Design review of the part built by this model. Coordinates are the model's own, in mm. Give positions to 0.01 mm unless a question says otherwise; leave off trailing zeros. Write each loop counter-clockwise with the first axis right and the second up, starting at its lowest first coordinate (ties: lowest second). Pieces come first, ordered by that corner, then holes. Notation, with made-up numbers: M 71,-26.5 L 75,-26.5 A25 cw 75,0.5 Z; hole C 10,73 d11. An arc over 180 degrees is marked long. Write each question's results on one line, items separated by ' | '. Start each with the question number.
from build123d import *

# Parameters (mm, degrees)
SKETCH1_R                    = 152.9969
SKETCH1_R_2                  = 123.825
BOSS_EXTRUDE1_DEPTH          = 22.352
SKETCH2_R                    = 127.254
CUT_EXTRUDE1_DEPTH           = 11.938
CHAMFER1_SIZE                = 0.762
SKETCH3_R                    = 4.2164
CUT_EXTRUDE2_DEPTH           = 23.352
CHAMFER2_SIZE                = 0.381
CIRPATTERN1_COUNT            = 32
CHAMFER2_OF_CIRPATTERN1_SIZE = 0.381
CUT_EXTRUDE3_DEPTH           = 0.79375


with BuildPart() as part:
    # Sketch1 → Boss-Extrude1 (new body)
    with BuildSketch(Plane(origin=(0, 0, 0), x_dir=(1, 0, 0), z_dir=(0, 1, 0))):
        Circle(SKETCH1_R)
        Circle(SKETCH1_R_2, mode=Mode.SUBTRACT)
    extrude(amount=BOSS_EXTRUDE1_DEPTH)

    # Sketch2 → Cut-Extrude1 (cut)
    with BuildSketch(Plane(origin=(0, 22.352, 0), x_dir=(-1, 0, 0), z_dir=(0, -1, 0))):
        Circle(SKETCH2_R)
    extrude(amount=CUT_EXTRUDE1_DEPTH, mode=Mode.SUBTRACT)

    # Chamfer1
    chamfer1_edges = [part.edges().sort_by_distance(p)[0] for p in [
        (127.254, 22.352, 0),
        (-152.9969, 0, 0),
        (-152.9969, 22.352, 0),
    ]]
    chamfer(chamfer1_edges, length=CHAMFER1_SIZE)

    # Sketch4 → Cut-Revolve1 (revolve, cut)
    with BuildSketch(Plane.XY):
        Polygon((-137.16, 0), (-137.16, 1.6256), (-134.366, 0.6604), (-134.366, 1.27), (0, 1.27), (0, 0), align=None)
    revolve(axis=Axis((0, 22.352, 0), (0, -1, 0)), mode=Mode.SUBTRACT)

    # Sketch3 → Cut-Extrude2 (cut, through all)
    with BuildSketch(Plane(origin=(0, 22.352, 0), x_dir=(1, 0, 0), z_dir=(0, 1, 0))):
        with Locations((-13.918306505, 141.314937447)):
            Circle(SKETCH3_R)
    cut_extrude2 = extrude(amount=-CUT_EXTRUDE2_DEPTH, mode=Mode.SUBTRACT)

    # Chamfer2
    chamfer2_edges = [part.edges().sort_by_distance(p)[0] for p in [
        (-18.134706505, 0, -141.314937447),
        (-18.134706505, 22.352, -141.314937447),
    ]]
    chamfer(chamfer2_edges, length=CHAMFER2_SIZE)

    # CirPattern1: Cut-Extrude2 ×32 about axis
    cirpattern1_axis = Axis((0, 0, 0), (0, 1, 0))
    for i in range(1, CIRPATTERN1_COUNT):
        add(cut_extrude2.rotate(cirpattern1_axis, i * 360 / CIRPATTERN1_COUNT), mode=Mode.SUBTRACT)

    # Chamfer2 of CirPattern1
    chamfer2_of_cirpattern1_edges = [part.edges().sort_by_distance(p)[0] for p in [
        (-45.355429856, 0, -135.061704818),
        (-45.355429856, 22.352, -135.061704818),
        (-70.833169474, 0, -123.618126616),
        (-70.833169474, 22.352, -123.618126616),
        (-93.588830113, 0, -107.423973133),
        (-93.588830113, 22.352, -107.423973133),
        (-112.747924496, 0, -87.101576608),
        (-112.747924496, 22.352, -87.101576608),
        (-127.57417937, 0, -63.43191534),
        (-127.57417937, 22.352, -63.43191534),
        (-137.497830076, 0, -37.324601139),
        (-137.497830076, 22.352, -37.324601139),
        (-142.137516281, 0, -9.782923448),
        (-142.137516281, 22.352, -9.782923448),
        (-141.314937447, 0, 18.134706505),
        (-141.314937447, 22.352, 18.134706505),
        (-135.061704818, 0, 45.355429856),
        (-135.061704818, 22.352, 45.355429856),
        (-123.618126616, 0, 70.833169474),
        (-123.618126616, 22.352, 70.833169474),
        (-107.423973133, 0, 93.588830113),
        (-107.423973133, 22.352, 93.588830113),
        (-87.101576608, 0, 112.747924496),
        (-87.101576608, 22.352, 112.747924496),
        (-63.43191534, 0, 127.57417937),
        (-63.43191534, 22.352, 127.57417937),
        (-37.324601139, 0, 137.497830076),
        (-37.324601139, 22.352, 137.497830076),
        (-9.782923448, 0, 142.137516281),
        (-9.782923448, 22.352, 142.137516281),
        (18.134706505, 0, 141.314937447),
        (18.134706505, 22.352, 141.314937447),
        (45.355429856, 0, 135.061704818),
        (45.355429856, 22.352, 135.061704818),
        (70.833169474, 0, 123.618126616),
        (70.833169474, 22.352, 123.618126616),
        (93.588830113, 0, 107.423973133),
        (93.588830113, 22.352, 107.423973133),
        (112.747924496, 0, 87.101576608),
        (112.747924496, 22.352, 87.101576608),
        (127.57417937, 0, 63.43191534),
        (127.57417937, 22.352, 63.43191534),
        (137.497830076, 0, 37.324601139),
        (137.497830076, 22.352, 37.324601139),
        (142.137516281, 0, 9.782923448),
        (142.137516281, 22.352, 9.782923448),
        (141.314937447, 0, -18.134706505),
        (141.314937447, 22.352, -18.134706505),
        (135.061704818, 0, -45.355429856),
        (135.061704818, 22.352, -45.355429856),
        (123.618126616, 0, -70.833169474),
        (123.618126616, 22.352, -70.833169474),
        (107.423973133, 0, -93.588830113),
        (107.423973133, 22.352, -93.588830113),
        (87.101576608, 0, -112.747924496),
        (87.101576608, 22.352, -112.747924496),
        (63.43191534, 0, -127.57417937),
        (63.43191534, 22.352, -127.57417937),
        (37.324601139, 0, -137.497830076),
        (37.324601139, 22.352, -137.497830076),
        (9.782923448, 0, -142.137516281),
        (9.782923448, 22.352, -142.137516281),
    ]]
    chamfer(chamfer2_of_cirpattern1_edges, length=CHAMFER2_OF_CIRPATTERN1_SIZE)

    # Sketch5 → Cut-Extrude3 (cut, symmetric)
    with BuildSketch(Plane.XY):
        Polygon((-135.676131126, 0.888656944), (-152.9969, 1.796399976), (-152.9969, -6.22182779), (-135.676131126, -6.22182779), align=None)
        Polygon((135.676131126, 0.888656944), (135.676131126, -6.22182779), (152.9969, -6.22182779), (152.9969, 1.796399976), align=None)
    extrude(amount=CUT_EXTRUDE3_DEPTH, both=True, mode=Mode.SUBTRACT)


solid = part.part
Q1. We need section A-A on x = 0. Write out the cut boundary in (y, z) (3 decimals).
Q2. Wall thickness on line 1 along Z through (x, y) = (-108, 15.25); line 2 along Z through (x, y) = (86.5, 20.5); line 3 along X through (y, z) = (17, -133): over which ranges is each line inside the solid? List them lowest first. Write a range as from..to.
Q3. For pin 1 Ø3 at (x, y) = (-11, 6.5) entering from +Z; pin 2 Ø4 at (y, z) = (17, -58.5) entering from +X; pin 3 Ø10 at (y, z) = (12.5, -116) entering from -X, all flat-tipped, find the tip position at first contact; note any pin that passes through.
Q4. The part is to be moulded in two halves that separate along X. For faces 1 (the cylindrical face through (-144.36, 11.327, -16.835)), 2 (the flat face through (-119, 1.27, 39)), 3 (the cylindrical face through (-33.17, 11.03, 149.36)), say which applies: pulls with the +X half, pulls with the -X half, needs draft (parallel to the pull), parting line crosses it, or undercut.
Answer sheet:
1) outline: M 0,-152.235 L 0.762,-152.997 L 21.59,-152.997 L 22.352,-152.235 L 22.352,-128.016 L 21.59,-127.254 L 10.414,-127.254 L 10.414,-123.825 L 1.27,-123.825 L 1.27,-134.366 L 0.66,-134.366 L 1.626,-137.16 L 0,-137.16 Z; M 0,137.16 L 1.626,137.16 L 0.66,134.366 L 1.27,134.366 L 1.27,123.825 L 10.414,123.825 L 10.414,127.254 L 21.59,127.254 L 22.352,128.016 L 22.352,152.235 L 21.59,152.997 L 0.762,152.997 L 0,152.235 Z
2) line 1: -108.37..-93.91, -86.25..-67.3, 67.3..86.25, 93.91..108.37 | line 2: -126.2..-111.99, -107.54..-93.33, 93.33..107.54, 111.99..126.2 | line 3: -75.62..-44.3, -38.14..38.14, 44.3..75.62
3) pin 1: z = 152.7 | pin 2: x = 142.18 | pin 3: x = -105.3
4) face 1: undercut | face 2: undercut | face 3: parting line crosses it
